The model under review builds one solid part; all positions refer to its coordinate system, in mm. A direction names the side the tool comes from. Give positions to 0.01 mm unless a question says otherwise; leave off trailing zeros. Loops run counter-clockwise (first coordinate to the right, second up) from the corner with the lowest first, then second, coordinate; pieces in that order, holes last. Notation, with made-up numbers: M 46,3.25 L 62,3.25 A8 cw 62,10.25 Z; hole C -8.75,19.5 d8. An arc over 180 degrees is marked long. Put each result on its own line as item: value. Start each with the question number.
```python
from build123d import *

# Parameters (mm, degrees)
VOLUME_BOITIER_DEPTH     = 90
ESQUISSE2_W              = 75
ESQUISSE2_H              = 60
FACE_INF_RIEURE_DEPTH    = 5
ESQUISSE3_W              = 5
ESQUISSE3_H              = 60
FACE_PILE_DEPTH          = 24
ENL_V_MAT_EXTRU_6_REACH  = 137.093
ESQUISSE11_R             = 3.5
ESQUISSE11_R_2           = 1.5
ESQUISSE12_W             = 3
ESQUISSE12_H             = 2
BOSS_EXTRU_7_DEPTH       = 85
ESQUISSE13_R             = 1.5
ESQUISSE13_R_2           = 1.527028633
ENL_V_MAT_EXTRU_7_DEPTH  = 20
ESQUISSE14_W             = 10
ESQUISSE14_H             = 5
ENL_V_MAT_EXTRU_8_DEPTH  = 5
ENL_V_MAT_EXTRU_9_REACH  = 129.475
ESQUISSE15_R             = 1.1
ENL_V_MAT_EXTRU_10_DEPTH = 90
ESQUISSE17_W             = 5
ESQUISSE17_H             = 5
ENL_V_MAT_EXTRU_11_DEPTH = 5
ESQUISSE18_W             = 2.3
ESQUISSE18_H             = 2.5
ENL_V_MAT_EXTRU_12_DEPTH = 5
ENL_V_MAT_EXTRU_13_REACH = 137.093
ESQUISSE20_W             = 15
ESQUISSE20_H             = 15
ENL_V_MAT_EXTRU_14_REACH = 129.475
ESQUISSE21_W             = 15
ESQUISSE21_H             = 10
ESQUISSE22_R             = 1.5
ENL_V_MAT_EXTRU_15_DEPTH = 10


with BuildPart() as part:
    # Esquisse1 → volume boitier (new body)
    with BuildSketch(Plane.XY):
        Polygon((0, 60), (0, 0), (7, 0), (7, 55), (70, 55), (70, 0), (75, 0), (75, 60), align=None)
    extrude(amount=VOLUME_BOITIER_DEPTH)

    # Esquisse2 → face inférieure (add)
    with BuildSketch(Plane.XY.offset(90)):
        with Locations((37.5, 30)):
            Rectangle(ESQUISSE2_W, ESQUISSE2_H)
    extrude(amount=FACE_INF_RIEURE_DEPTH)

    # Esquisse3 → face pile (add)
    with BuildSketch(Plane(origin=(0, 0, 0), x_dir=(-1, 0, 0), z_dir=(0, 0, -1))):
        with Locations((-72.5, 30)):
            Rectangle(ESQUISSE3_W, ESQUISSE3_H)
    extrude(amount=FACE_PILE_DEPTH)

    # Esquisse11 → Enlèv. mat.-Extru.6 (cut, up to next)
    with BuildSketch(Plane(origin=(75, 0, 0), x_dir=(0, 0, -1), z_dir=(1, 0, 0)), mode=Mode.PRIVATE) as enl_v_mat_extru_6_sk1:
        with Locations((-16, 30)):
            Circle(ESQUISSE11_R)
    enl_v_mat_extru_6_tool1 = extrude(enl_v_mat_extru_6_sk1.sketch, amount=-ENL_V_MAT_EXTRU_6_REACH, mode=Mode.PRIVATE) & part.part
    # Esquisse11 → Enlèv. mat.-Extru.6 (cut, up to next)
    with BuildSketch(Plane(origin=(75, 0, 0), x_dir=(0, 0, -1), z_dir=(1, 0, 0)), mode=Mode.PRIVATE) as enl_v_mat_extru_6_sk2:
        with Locations((-87.5, 2.5)):
            Circle(ESQUISSE11_R_2)
    enl_v_mat_extru_6_tool2 = extrude(enl_v_mat_extru_6_sk2.sketch, amount=-ENL_V_MAT_EXTRU_6_REACH, mode=Mode.PRIVATE) & part.part
    add(enl_v_mat_extru_6_tool1.solids().sort_by_distance((75, 30, 16))[0], mode=Mode.SUBTRACT)
    add(enl_v_mat_extru_6_tool2.solids().sort_by_distance((75, 2.5, 87.5))[0], mode=Mode.SUBTRACT)

    # Esquisse12 → Boss.-Extru.7 (add)
    with BuildSketch(Plane(origin=(0, 0, 90), x_dir=(-1, 0, 0), z_dir=(0, 0, -1))):
        Polygon((-70, 20), (-70, 23), (-27, 23), (-27, 15), (-29, 15), (-29, 20), align=None)
        with Locations((-68.5, 6)):
            Rectangle(ESQUISSE12_W, ESQUISSE12_H)
        with Locations((-8.5, 6)):
            Rectangle(ESQUISSE12_W, ESQUISSE12_H)
    extrude(amount=BOSS_EXTRU_7_DEPTH)

    # Esquisse13 → Enlèv. mat.-Extru.7 (cut)
    with BuildSketch(Plane.ZY):
        with Locations((2.5, 2.5)):
            Circle(ESQUISSE13_R)
        with Locations((2.5, 57.5)):
            Circle(ESQUISSE13_R_2)
    extrude(amount=-ENL_V_MAT_EXTRU_7_DEPTH, mode=Mode.SUBTRACT)

    # Esquisse14 → Enlèv. mat.-Extru.8 (cut)
    with BuildSketch(Plane(origin=(0, 0, 0), x_dir=(-1, 0, 0), z_dir=(0, 0, -1))):
        with Locations((-65, 57.5)):
            Rectangle(ESQUISSE14_W, ESQUISSE14_H)
        with Locations((-12, 57.5)):
            Rectangle(ESQUISSE14_W, ESQUISSE14_H)
    extrude(amount=-ENL_V_MAT_EXTRU_8_DEPTH, mode=Mode.SUBTRACT)

    # Esquisse15 → Enlèv. mat.-Extru.9 (cut, up to next)
    with BuildSketch(Plane.XZ.offset(-20), mode=Mode.PRIVATE) as enl_v_mat_extru_9_sk1:
        with Locations((33, 70)):
            Circle(ESQUISSE15_R)
    enl_v_mat_extru_9_tool1 = extrude(enl_v_mat_extru_9_sk1.sketch, amount=-ENL_V_MAT_EXTRU_9_REACH, mode=Mode.PRIVATE) & part.part
    add(enl_v_mat_extru_9_tool1.solids().sort_by_distance((33, 20, 70))[0], mode=Mode.SUBTRACT)

    # Esquisse16 → Enlèv. mat.-Extru.10 (cut)
    with BuildSketch(Plane.XY.offset(95)):
        Polygon((0, 2.5), (2.3, 2.5), (2.3, 5), (5, 5), (5, 0), (0, 0), align=None)
        Polygon((0, 60), (0, 57.5), (2.3, 57.5), (2.3, 55), (5, 55), (5, 60), align=None)
    extrude(amount=-ENL_V_MAT_EXTRU_10_DEPTH, mode=Mode.SUBTRACT)

    # Esquisse17 → Enlèv. mat.-Extru.11 (cut)
    with BuildSketch(Plane.ZY):
        with Locations((2.5, 2.5)):
            Rectangle(ESQUISSE17_W, ESQUISSE17_H)
        with Locations((2.5, 57.5)):
            Rectangle(ESQUISSE17_W, ESQUISSE17_H)
    extrude(amount=-ENL_V_MAT_EXTRU_11_DEPTH, mode=Mode.SUBTRACT)

    # Esquisse18 → Enlèv. mat.-Extru.12 (cut)
    with BuildSketch(Plane.XY.offset(95)):
        with Locations((1.15, 3.75)):
            Rectangle(ESQUISSE18_W, ESQUISSE18_H)
        with Locations((1.15, 56.25)):
            Rectangle(ESQUISSE18_W, ESQUISSE18_H)
    extrude(amount=-ENL_V_MAT_EXTRU_12_DEPTH, mode=Mode.SUBTRACT)

    # Esquisse20 → Enlèv. mat.-Extru.13 (cut, up to next)
    with BuildSketch(Plane.ZY, mode=Mode.PRIVATE) as enl_v_mat_extru_13_sk1:
        with Locations((27.5, 30)):
            Rectangle(ESQUISSE20_W, ESQUISSE20_H)
    enl_v_mat_extru_13_tool1 = extrude(enl_v_mat_extru_13_sk1.sketch, amount=-ENL_V_MAT_EXTRU_13_REACH, mode=Mode.PRIVATE) & part.part
    # Esquisse20 → Enlèv. mat.-Extru.13 (cut, up to next)
    with BuildSketch(Plane.ZY, mode=Mode.PRIVATE) as enl_v_mat_extru_13_sk2:
        with Locations((67.5, 30)):
            Rectangle(ESQUISSE20_W, ESQUISSE20_H)
    enl_v_mat_extru_13_tool2 = extrude(enl_v_mat_extru_13_sk2.sketch, amount=-ENL_V_MAT_EXTRU_13_REACH, mode=Mode.PRIVATE) & part.part
    add(enl_v_mat_extru_13_tool1.solids().sort_by_distance((0, 30, 27.5))[0], mode=Mode.SUBTRACT)
    add(enl_v_mat_extru_13_tool2.solids().sort_by_distance((0, 30, 67.5))[0], mode=Mode.SUBTRACT)

    # Esquisse21 → Enlèv. mat.-Extru.14 (cut, up to next)
    with BuildSketch(Plane.XZ.offset(-20), mode=Mode.PRIVATE) as enl_v_mat_extru_14_sk1:
        with Locations((49.5, 67)):
            Rectangle(ESQUISSE21_W, ESQUISSE21_H)
    enl_v_mat_extru_14_tool1 = extrude(enl_v_mat_extru_14_sk1.sketch, amount=-ENL_V_MAT_EXTRU_14_REACH, mode=Mode.PRIVATE) & part.part
    add(enl_v_mat_extru_14_tool1.solids().sort_by_distance((49.5, 20, 67))[0], mode=Mode.SUBTRACT)

    # Esquisse22 → Enlèv. mat.-Extru.15 (cut)
    with BuildSketch(Plane.XZ.offset(-5)):
        with Locations(Location((2.5, 92.5, 0), (0, 0, 270))):
            Circle(ESQUISSE22_R)
    extrude(amount=-ENL_V_MAT_EXTRU_15_DEPTH, mode=Mode.SUBTRACT)


solid = part.part
```
Item 1: Tool access review of faces 1 (the flat face through (70, 30, 34)), 2 (the flat face through (3, 22.5, 67)), 3 (the flat face through (69, 5, 48)): name each direction out of +Z, -Z, +X, -X, +Y, -Y from which nothing blocks a thin tool from reaching the whole face with its end or side.
Item 2: Consider section A-A, the plane x = 39. Write out the cut boundary in (y, z).
Item 3: To check wall thickness, follow L1, parallel to X at y = 21.3, z = 70; L2, parallel to Y at x = 6.05, z = 2.5; L3, parallel to Y at x = 18.9, z = 2.5. State the ranges of each line that lie inside material, in increasing order. Write a range as [from, to].
Item 4: Consider section B-B, the plane y = 53. Write out the cut boundary in (x, z).
Item 5: Draft analysis for pull direction Z (two halves, no side actions). For faces 4 (the flat face through (37, 30, 95)), 5 (the flat face through (3, 30, 35)), 6 (the flat face through (60, 57, 2)), state which applies: +Z half, -Z half, draft (parallel to the pull), parting line (faces both ways), or undercut.
Item 6: Clearance check with flat-ended pins moving along their axes: pin 1 Ø3 at (x, z) = (17, 78.5) entering from -Y; pin 2 Ø1.5 at (x, y) = (47.5, 21.5) entering from -Z; pin 3 Ø2.5 at (y, z) = (2.5, 2.5) entering from -X. State where each tip first meets the part, or that it passes through.
Item 7: Consider section C-C, the plane x = 55.5. Write out the cut boundary in (y, z).
Report:
1. face 1: -Z
1. face 2: -X
1. face 3: -Z, -Y
2. outline: M 0,90 L 20,90 L 20,5 L 23,5 L 23,90 L 55,90 L 55,0 L 60,0 L 60,95 L 0,95 Z
3. L1: [0, 7], [27, 31.9], [34.1, 42], [57, 75]
3. L2: [0, 1], [4, 55.97], [59.03, 60]
3. L3: [55, 55.97], [59.03, 60]
4. outline: M 0,0 L 7,0 L 7,90 L 70,90 L 70,-24 L 75,-24 L 75,95 L 0,95 Z
5. face 4: +Z half
5. face 5: undercut
5. face 6: draft
6. pin 1: y = 55
6. pin 2: z = 5
6. pin 3: x = 70
7. outline: M 0,90 L 20,90 L 20,72 L 23,72 L 23,90 L 55,90 L 55,0 L 60,0 L 60,95 L 0,95 Z; M 20,5 L 23,5 L 23,62 L 20,62 Z
